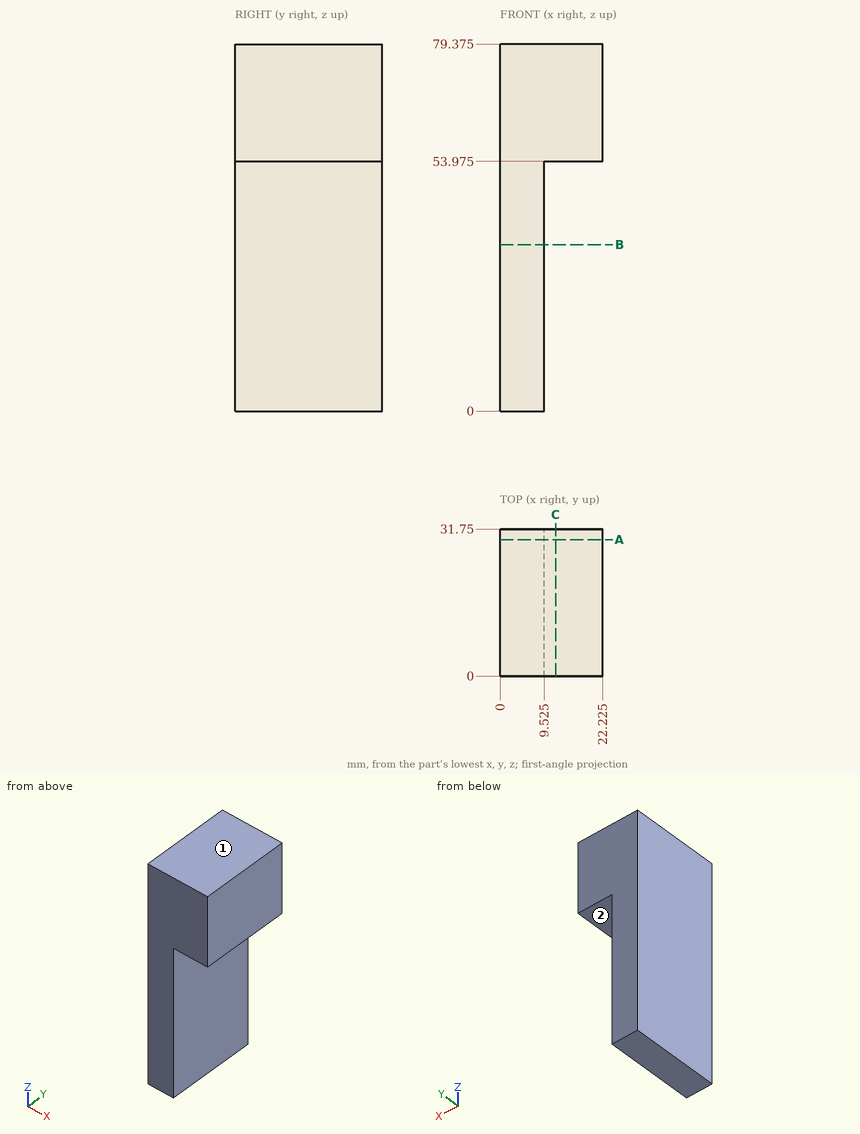
Design review of the part shown in the three views and the two pictorial views. Dimensions are in mm from the part's minimum x, y and z. A direction names the side the tool comes from. Coordinates: 2 decimals unless noted, no trailing zeros. Order: outer loops, then holes, each group sorted by start corner. A loop starts at its lowest first (then second) coordinate and runs counter-clockwise, first axis right, second up.
1) Take a section at B-B, the plane z = 36. Give the boundary of the cut face in (x, y) (3 decimals), and give its area (3 significant figures).
2) Clearance check with a flat-ended pin moving along its axis: pin 1 (10 mm diameter, centred on x = 15.5, y = 12.5, fed in from -Z) (3 decimals). State where the tip first meets the part, or that it passes through.
3) Wall thickness on line 1 along Z through (x, y) = (19, 29.5) (3 decimals); line 2 along X through (y, z) = (7, 7) (3 decimals): over which ranges is each line inside the solid? List them lowest first.
4) Take a section at A-A, the plane y = 29.5. Give the boundary of the cut face in (x, z) (3 decimals), and give its area (3 significant figures).
5) For the marked faces 1 and 2, list the 3-axis set-ups (+Z, -Z, +X, -X, +Y, -Y) from which the entire face can be reached by the end or side of a thin tool; tool diameter is ignored.
6) Take a section at C-C, the plane x = 12. Give the boundary of the cut face in (y, z) (3 decimals).
Returned:
1. outline: (0, 0) - (9.525, 0) - (9.525, 31.75) - (0, 31.75) - close
1. area: 302 mm2
2. pin 1: stops at z = 53.975
3. line 1: z = 53.975 to 79.375
3. line 2: x = 0 to 9.525
4. outline: (0, 0) - (9.525, 0) - (9.525, 53.975) - (22.225, 53.975) - (22.225, 79.375) - (0, 79.375) - close
4. area: 1,080 mm2
5. face 1: +Z, +X, -X, +Y, -Y
5. face 2: -Z, +X, +Y, -Y
6. outline: (0, 53.975) - (31.75, 53.975) - (31.75, 79.375) - (0, 79.375) - close
